Geometry: final body of the model. Coordinates: model frame, mm. Face numbers are marked on the shaded views. Give positions to 0.01 mm unless a question says otherwise; leave off trailing zeros. Order: outer loops, then holes, each group sorted by start corner. A loop starts at its lowest first (then second) coordinate and runs counter-clockwise, first axis right, second up. Notation, with made-up numbers: M 19,6 L 64,6 A29 ccw 64,37 Z; hole C 50.25,18.5 d5. An arc over 180 degrees is marked long. Write item = value, one per line. Start each with the question number.
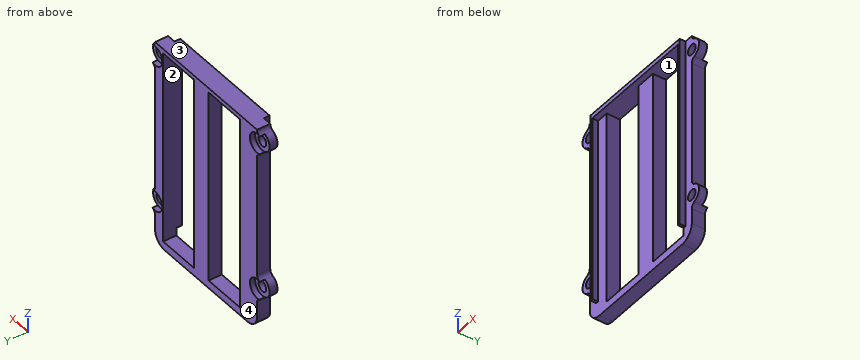
from build123d import *

# Parameters (mm, degrees)
SKETCH2_R           = 2
BOSS_EXTRUDE1_DEPTH = 3
BOSS_EXTRUDE2_DEPTH = 2
FILLET1_R           = 5
SKETCH4_W           = 16
SKETCH4_H           = 74.3
SKETCH4_W_2         = 16.4
CUT_EXTRUDE1_DEPTH  = 10
BOSS_EXTRUDE3_DEPTH = 2.2


with BuildPart() as part:
    # Sketch2 → Boss-Extrude1 (new body)
    with BuildSketch(Plane(origin=(0, 0, 0), x_dir=(1, 0, 0), z_dir=(0, 1, 0))):
        with BuildLine():
            Line((57.160001108, 49.763863032), (4.160001108, 49.763863032))
            Line((4.160001108, 49.763863032), (4.160001108, 38.892058935))
            ThreePointArc((4.160001108, 38.892058935), (3.801845246, 37.749978453), (2.855653282, 37.016940791))
            ThreePointArc((2.855653282, 37.016940791), (0.410001108, 33.501094271), (2.855653282, 29.985247752))
            ThreePointArc((2.855653282, 29.985247752), (3.801845246, 29.25221009), (4.160001108, 28.110129608))
            Line((4.160001108, 28.110129608), (4.160001108, -18.486673333))
            ThreePointArc((4.160001108, -18.486673333), (3.801845246, -19.628753814), (2.855653282, -20.361791477))
            ThreePointArc((2.855653282, -20.361791477), (0.410001109, -23.877730206), (2.855826188, -27.393548657))
            ThreePointArc((2.855826188, -27.393548657), (3.792729548, -28.113251523), (4.160001108, -29.236136968))
            Line((4.160001108, -29.236136968), (7.160001108, -29.236136968))
            Line((7.160001108, -29.236136968), (54.160001108, -29.236136968))
            Line((54.160001108, -29.236136968), (57.160001108, -29.236136968))
            ThreePointArc((57.160001108, -29.236136968), (57.527272669, -28.113251523), (58.464176029, -27.393548657))
            ThreePointArc((58.464176029, -27.393548657), (60.910001107, -23.877730206), (58.464348934, -20.361791477))
            ThreePointArc((58.464348934, -20.361791477), (57.51815697, -19.628753814), (57.160001108, -18.486673333))
            Line((57.160001108, -18.486673333), (57.160001108, 28.110129608))
            ThreePointArc((57.160001108, 28.110129608), (57.51815697, 29.25221009), (58.464348934, 29.985247752))
            ThreePointArc((58.464348934, 29.985247752), (60.910001108, 33.501094271), (58.464348934, 37.016940791))
            ThreePointArc((58.464348934, 37.016940791), (57.51815697, 37.749978453), (57.160001108, 38.892058935))
            Line((57.160001108, 38.892058935), (57.160001108, 49.763863032))
        make_face()
        with Locations(Location((4.160001108, 33.501094271, 0), (0, 0, 270))):
            Circle(SKETCH2_R, mode=Mode.SUBTRACT)
        with Locations(Location((57.160001108, 33.501094271, 0), (0, 0, 270))):
            Circle(SKETCH2_R, mode=Mode.SUBTRACT)
        with Locations(Location((57.160001108, -23.877637996, 0), (0, 0, 270))):
            Circle(SKETCH2_R, mode=Mode.SUBTRACT)
        with Locations(Location((4.160001108, -23.877637996, 0), (0, 0, 270))):
            Circle(SKETCH2_R, mode=Mode.SUBTRACT)
    extrude(amount=BOSS_EXTRUDE1_DEPTH)

    # Sketch3 → Boss-Extrude2 (add)
    with BuildSketch(Plane(origin=(0, 3, 0), x_dir=(1, 0, 0), z_dir=(0, 1, 0))):
        with BuildLine():
            Line((57.160001108, 38.892058935), (57.160001108, 49.763863032))
            Line((57.160001108, 49.763863032), (4.160001108, 49.763863032))
            Line((4.160001108, 49.763863032), (4.160001108, 38.892058935))
            ThreePointArc((4.160001108, 38.892058935), (3.801845246, 37.749978453), (2.855653282, 37.016940791))
            ThreePointArc((2.855653282, 37.016940791), (7.910001108, 33.501094271), (2.855653282, 29.985247752))
            ThreePointArc((2.855653282, 29.985247752), (3.801845246, 29.25221009), (4.160001108, 28.110129608))
            Line((4.160001108, 28.110129608), (4.160001108, -18.486673333))
            ThreePointArc((4.160001108, -18.486673333), (3.801845246, -19.628753814), (2.855653282, -20.361791477))
            ThreePointArc((2.855653282, -20.361791477), (7.910001107, -23.877545787), (2.855826188, -27.393548657))
            ThreePointArc((2.855826188, -27.393548657), (3.792729548, -28.113251523), (4.160001108, -29.236136968))
            Line((4.160001108, -29.236136968), (57.160001108, -29.236136968))
            ThreePointArc((57.160001108, -29.236136968), (57.527272669, -28.113251523), (58.464176029, -27.393548657))
            ThreePointArc((58.464176029, -27.393548657), (53.410001109, -23.877545787), (58.464348934, -20.361791477))
            ThreePointArc((58.464348934, -20.361791477), (57.51815697, -19.628753814), (57.160001108, -18.486673333))
            Line((57.160001108, -18.486673333), (57.160001108, 28.110129608))
            ThreePointArc((57.160001108, 28.110129608), (57.51815697, 29.25221009), (58.464348934, 29.985247752))
            ThreePointArc((58.464348934, 29.985247752), (53.410001108, 33.501094271), (58.464348934, 37.016940791))
            ThreePointArc((58.464348934, 37.016940791), (57.51815697, 37.749978453), (57.160001108, 38.892058935))
        make_face()
    extrude(amount=BOSS_EXTRUDE2_DEPTH)

    # Fillet1
    fillet1_edges = [part.edges().sort_by_distance(p)[0] for p in [
        (4.160001108, 2.5, -49.763863032),
        (57.160001108, 2.5, -49.763863032),
    ]]
    fillet(fillet1_edges, radius=FILLET1_R)

    # Sketch4 → Cut-Extrude1 (cut)
    with BuildSketch(Plane(origin=(0, 5, 0), x_dir=(1, 0, 0), z_dir=(0, 1, 0))):
        with Locations((44.960001108, 9.613863032)):
            Rectangle(SKETCH4_W, SKETCH4_H)
        with Locations((21.160001108, 9.613863032)):
            Rectangle(SKETCH4_W_2, SKETCH4_H)
    extrude(amount=-CUT_EXTRUDE1_DEPTH, mode=Mode.SUBTRACT)

    # Sketch7 → Boss-Extrude3 (add)
    with BuildSketch(Plane.XZ):
        Polygon((53.860001108, 29.236136968), (53.860001108, -43.805670275), (52.960001108, -43.805670275), (52.960001108, 27.536136968), (8.460001108, 27.536136968), (8.460001108, -43.805670275), (7.460001108, -43.805670275), (7.460001108, 29.236136968), align=None)
    extrude(amount=BOSS_EXTRUDE3_DEPTH)


solid = part.part
1) Ray query, L1, parallel to X at y = 4.25, z = -39; L2, parallel to Z at x = 14.5, y = 2.25; L3, parallel to X at y = -0.5, z = 2. Return the intervals inside material, ascending.
2) Draft query along Z for the marked faces 1, 2, 3 and 4. Return one class per face: pulls with the +Z half, pulls with the -Z half, needs draft (parallel to the pull), parting line crosses it, or undercut.
3) Pin query (flat end, axial travel): pin 1 Ø1.5 at (y, z) = (2.5, -40.5) entering from -X; pin 2 Ø2 at (y, z) = (0.5, -27.5) entering from -X; pin 3 Ø2.5 at (y, z) = (3.5, -16) entering from +X; pin 4 Ø8.5 at (x, z) = (57.16, -33.5) entering from +Y. Return the tip coordinate at first contact, or that it passes through.
4) Cut plane B-B (z = -4). Return loops of the section in (x, y).
5) Cut plane D-D (y = -1). Return loops of the section in (x, z), plus the area to 3 significant figures.
6) Cut plane A-A (z = -33.5). Give the number of separate pieces and of enclosed holes in the cut face, plus the area to 3 significant figures.
7) Cut plane C-C (x = 48). Return loops of the section in (y, z), plus the area to 3 significant figures.
Reply:
q1.L1 = 4.16 to 12.96, 29.36 to 36.96, 52.96 to 57.16
q1.L2 = -49.76 to -46.76, 27.54 to 29.24
q1.L3 = 7.46 to 8.46, 52.96 to 53.86
q2.face_1 = undercut
q2.face_2 = undercut
q2.face_3 = pulls with the +Z half
q2.face_4 = needs draft
q3.pin_1 = 4.16
q3.pin_2 = 4.12
q3.pin_3 = 57.16
q3.pin_4 = 5
q4.outline = M 4.16,0 L 7.46,0 L 7.46,-2.2 L 8.46,-2.2 L 8.46,0 L 12.96,0 L 12.96,5 L 4.16,5 Z; M 29.36,0 L 36.96,0 L 36.96,5 L 29.36,5 Z; M 52.96,-2.2 L 53.86,-2.2 L 53.86,0 L 57.16,0 L 57.16,5 L 52.96,5 Z
q5.outline = M 7.46,-43.81 L 8.46,-43.81 L 8.46,27.54 L 52.96,27.54 L 52.96,-43.81 L 53.86,-43.81 L 53.86,29.24 L 7.46,29.24 Z
q5.area = 214 mm²
q6.separate_pieces = 5
q6.enclosed_holes = 0
q6.area = 90.7 mm²
q7.outline = M -2.2,27.54 L 5,27.54 L 5,29.24 L -2.2,29.24 Z; M 0,-49.76 L 5,-49.76 L 5,-46.76 L 0,-46.76 Z
q7.area = 27.2 mm²
